Autodesk Inventor part; units mm, degrees
ref_plane "YZ Plane" through (0, 0, 0) normal (1, 0, 0) x (0, 1, 0)
ref_plane "XZ Plane" through (0, 0, 0) normal (0, 1, 0) x (-1, 0, 0)
ref_plane "XY Plane" through (0, 0, 0) normal (0, 0, 1) x (1, 0, 0)
sketch "Sketch1" plane through (0, 0, 0) normal (0, 0, 1) x (1, 0, 0)
  line L0 (0, 0) -> (69.85, 0)
  line L1 (69.85, 0) -> (69.85, 76.2)
  line L2 (0, 76.2) -> (0, 0)
  line L3 (64.77, 76.2) -> (64.77, 5.08)
  line L4 (64.77, 5.08) -> (5.08, 5.08)
  line L5 (5.08, 5.08) -> (5.08, 76.2)
  line L6 (69.85, 76.2) -> (64.77, 76.2)
  line L7 (5.08, 76.2) -> (0, 76.2)
  dimension "d0" = 69.85
  dimension "d1" = 5.08
  dimension "d2" = 5.08
  dimension "d3" = 76.2
extrude "Extrusion1" add sketch "Sketch1" along normal blind 25.4
sketch "Sketch2" plane through (0, 0, 0) normal (0, -1, 0) x (1, 0, 0)
  line L0 (22.225, 38.1) -> (47.625, 38.1)
  line L1 (47.625, 38.1) -> (47.625, -12.7)
  line L2 (47.625, -12.7) -> (22.225, -12.7)
  line L3 (22.225, -12.7) -> (22.225, 38.1)
  line L4 (0, 25.4) -> (69.85, 25.4) construction
  line L5 (0, 25.4) -> (22.225, 38.1) construction
  line L6 (0, 0) -> (69.85, 0) construction
  line L7 (0, 0) -> (22.225, -12.7) construction
  line L8 (47.625, 38.1) -> (69.85, 25.4) construction
  line L9 (47.625, -12.7) -> (69.85, 0) construction
  dimension "d6" = 50.8
  dimension "d7" = 25.4
extrude "Extrusion2" add sketch "Sketch2" against normal up to surface (5.08 mm away)
sketch "Sketch3" plane through (69.85, 0, 0) normal (0, -1, 0) x (1, 0, 0)
  line L0 (-22.225, 38.1) -> (-47.625, 38.1) construction
  line L1 (-47.425, 38.1) -> (-22.425, 38.1) construction
  line L2 (-22.425, 38.1) -> (-22.425, 14.238) construction
  line L3 (-22.425, 14.238) -> (-47.425, 14.238) construction
  line L4 (-47.425, 14.238) -> (-47.425, 38.1) construction
  line L5 (-5.08, 25.4) -> (-22.225, 25.4) construction
  line L6 (-22.225, 25.4) -> (-22.425, 25.4) construction
  line L7 (-69.85, 25.4) -> (-47.625, 25.4) construction
  line L8 (-47.625, 25.4) -> (-47.425, 25.4) construction
  circle A0 centre (-45.425, 16.238) radius 1.25
  circle A1 centre (-24.425, 16.238) radius 1.25
  circle A2 centre (-45.425, 28.738) radius 1.25
  circle A3 centre (-24.425, 28.738) radius 1.25
  line L9 (-39.425, 33.138) -> (-30.425, 33.138)
  line L10 (-30.425, 33.138) -> (-30.425, 24.138)
  line L11 (-30.425, 24.138) -> (-39.425, 24.138)
  line L12 (-39.425, 24.138) -> (-39.425, 33.138)
  line L13 (-39.425, 33.138) -> (-30.425, 24.138) construction
  line L14 (-39.425, 24.138) -> (-30.425, 33.138) construction
  point P0 (-69.85, 0)
  point P1 (-34.925, 28.638)
  dimension "d10" = 23.862
  dimension "d11" = 25
  dimension "d12" = 2.5
  dimension "d13" = 2
  dimension "d14" = 2
  dimension "d15" = 2
  dimension "d16" = 14.5
  dimension "d17" = 9
  dimension "d18" = 9.462
  dimension "d19" = 12.5
extrude "Extrusion3" cut sketch "Sketch3" against normal up to surface (5.08 mm away)
sketch "Sketch4" plane through (0, 0, 0) normal (0, -1, 0) x (1, 0, 0)
  line L0 (22.225, 0) -> (22.225, -12.7) construction
  line L1 (22.225, -12.7) -> (47.625, -12.7) construction
  line L2 (47.625, -12.7) -> (47.625, 12.7) construction
  line L3 (47.625, 12.7) -> (22.225, 12.7) construction
  line L4 (22.225, 12.7) -> (22.225, -12.7) construction
  line L5 (47.625, -12.7) -> (47.625, 0) construction
  line L6 (22.225, 12.7) -> (47.625, -12.7) construction
  line L7 (47.625, 12.7) -> (22.225, -12.7) construction
  line L8 (26.035, 8.89) -> (43.815, 8.89)
  line L9 (43.815, 8.89) -> (43.815, -8.89)
  line L10 (43.815, -8.89) -> (26.035, -8.89)
  line L11 (26.035, -8.89) -> (26.035, 8.89)
  circle A0 centre (24.765, 10.16) radius 1.25
  circle A1 centre (45.085, 10.16) radius 1.25
  circle A2 centre (45.085, -10.16) radius 1.25
  circle A3 centre (24.765, -10.16) radius 1.25
  point P0 (0, 0)
  dimension "d22" = 2.5
  dimension "d23" = 20.32
  dimension "d24" = 17.78
extrude "Extrusion4" cut sketch "Sketch4" against normal up to surface (5.08 mm away)
sketch "Sketch5" plane through (0, 0, 0) normal (-1, 0, 0) x (0, 0, 1)
  line L0 (0, 76.2) -> (25.4, 76.2) construction
  line L1 (0, 76.2) -> (0, 5.08) construction
  line L2 (25.4, 76.2) -> (0, 76.2) construction
  line L3 (0, 76.2) -> (0, 50.8) construction
  line L4 (0, 50.8) -> (25.4, 50.8) construction
  line L5 (25.4, 50.8) -> (25.4, 76.2) construction
  line L6 (25.4, 76.2) -> (0, 50.8) construction
  line L7 (25.4, 50.8) -> (0, 76.2) construction
  arc A0 (14.4861, 60.875) -> (10.9139, 60.875) centre (12.7, 63.5) ccw construction
  line L8 (14.4861, 60.875) -> (10.9139, 60.875) construction
  line L9 (10.8534, 60.675) -> (14.5466, 60.675)
  arc A1 (14.5466, 60.675) -> (10.8534, 60.675) centre (12.7, 63.5) ccw
  point P0 (0, 0)
  dimension "d27" = 25.4
  dimension "d28" = 6.35
  dimension "d29" = 5.8
  dimension "d54" = 0.2
extrude "Extrusion5" cut sketch "Sketch5" against normal up to surface (5.08 mm away)
sketch "Sketch6" plane through (69.85, 0, 0) normal (1, 0, 0) x (0, 0, -1)
  line L0 (-25.4, 76.2) -> (-25.4, 0) construction
  line L1 (-25.4, 76.2) -> (0, 50.8) construction
  line L2 (0, 76.2) -> (0, 0) construction
  line L3 (0, 76.2) -> (-25.4, 76.2) construction
  line L4 (0, 76.2) -> (-25.4, 50.8) construction
  line L5 (-25.4, 0) -> (-25.4, 76.2) construction
  line L6 (-25.4, 50.8) -> (0, 50.8) construction
  line L7 (-25.4, 5.08) -> (-25.4, 76.2)
  circle A0 centre (-12.7, 63.5) radius 2.6035
  dimension "d52" = 25.4
  dimension "d53" = 5.207
extrude "Extrusion6" cut sketch "Sketch6" against normal up to surface (5.08 mm away)
fillet "Fillet1" radius 2 4 edges at (47.625, 2.54, 38.1) (22.225, 2.54, 38.1) (22.225, 2.54, -12.7) (47.625, 2.54, -12.7)
fillet "Fillet2" radius 6.35 4 edges at (67.31, 76.2, 25.4) (67.31, 76.2, 0) (2.54, 76.2, 25.4) (2.54, 76.2, 0)
chamfer "Chamfer1" distance 6.35 angle 45 4 edges at (0, 0, 12.7) (5.08, 5.08, 12.7) (69.85, 0, 12.7) (64.77, 5.08, 12.7)
sketch "Sketch7" plane through (0, 76.2, 6.35) normal (-1, 0, 0) x (0, 0, 1)
  line L0 (12.7, -22.225) -> (0, -22.225)
  line L1 (0, -22.225) -> (0, -69.85)
  line L2 (0, -69.85) -> (12.7, -69.85)
  line L3 (12.7, -69.85) -> (12.7, -22.225)
  line L4 (-6.35, -6.35) -> (-6.35, -69.85)
  line L5 (19.05, -69.85) -> (-6.35, -69.85)
  line L6 (19.05, -6.35) -> (19.05, -69.85)
  arc A0 (8.975, -10.9139) -> (8.975, -14.4861) centre (6.35, -12.7) ccw
  point P0 (-6.35, -76.2)
  dimension "d42" = 6.35
  dimension "d43" = 0
  dimension "d44" = 6.35
  dimension "d46" = 6.35
extrude "Extrusion7" cut sketch "Sketch7" against normal through all
chamfer "Chamfer2" distance 3.175 angle 45 8 edges at (64.77, 6.35, 19.05) (64.77, 6.35, 6.35) (67.31, 53.975, 6.35) (67.31, 53.975, 19.05) (5.08, 6.35, 6.35) (5.08, 6.35, 19.05) (2.54, 53.975, 19.05) (2.54, 53.975, 6.35)
fillet "Fillet3" radius 3.175 4 edges at (26.035, 2.54, 8.89) (26.035, 2.54, -8.89) (43.815, 2.54, -8.89) (43.815, 2.54, 8.89)
sketch "Sketch8" plane through (0, 76.2, 6.35) normal (-1, 0, 0) x (0, 0, 1)
  arc A0 (8.1966, -15.525) -> (4.5034, -15.525) centre (6.35, -12.7) ccw
  line L0 (8.1966, -15.525) -> (4.5034, -15.525)
  arc A1 (8.6238, -17.125) -> (4.0762, -17.125) centre (6.35, -12.7) ccw
  line L1 (8.6238, -17.125) -> (4.0762, -17.125)
  point P0 (-6.35, -76.2)
  dimension "d56" = 1.6
extrude "Extrusion8" add sketch "Sketch8" along normal blind 4.525
sketch "Sketch9" plane through (5.08, 76.2, 19.05) normal (1, 0, 0) x (0, 0, -1)
  line L0 (8.1966, -15.525) -> (4.5034, -15.525)
  arc A0 (8.1966, -15.525) -> (4.5034, -15.525) centre (6.35, -12.7) ccw
  line L1 (4.0762, -17.125) -> (8.6238, -17.125)
  arc A1 (8.6238, -17.125) -> (4.0762, -17.125) centre (6.35, -12.7) ccw
  point P0 (19.05, -76.2)
  dimension "d59" = 1.6
extrude "Extrusion9" add sketch "Sketch9" along normal blind 5.4
sketch "Sketch10" plane through (69.85, 76.2, 19.05) normal (1, 0, 0) x (0, 0, -1)
  circle A0 centre (6.35, -12.7) radius 2.6035
  circle A1 centre (6.35, -12.7) radius 4.2035
  point P0 (19.05, -76.2)
  dimension "d62" = 1.6
extrude "Extrusion10" add sketch "Sketch10" along normal blind 2.54
properties part number "HoseMount"
Check sheet for the modelled part. Datum: model origin and axes. Units: mm. A direction names the side the tool comes from. Give positions to 0.01 mm unless a question says otherwise; leave off trailing zeros. Loops run counter-clockwise (first coordinate to the right, second up) from the corner with the lowest first, then second, coordinate; pieces in that order, holes last. Notation, with made-up numbers: (10, 23.5) - (14, 23.5) arc R17 ccw to (14, 47.5) - close; hole circle Ø9 at (18, -9). An arc over 180 degrees is marked (long way). One line per question, with ' | ' between items. Start each with the question number.
1. Material ranges on line 1 along X through (y, z) = (1, -10) (3 decimals); line 2 along Z through (x, y) = (0.5, 63.5); line 3 along X through (y, z) = (48.5, 22), recorded low to high. Write a range as [from, to].
2. Draft check along X on faces 6 (the flat face through (10.48, 65, 16)), 7 (the cylindrical face through (22.795, 2.576, 37.499)), 8 (the flat face through (35, 3, 8.89)), 9 (the flat face through (65.828, 7.96, 17.485)). Enter one of: released by +X, released by -X, zero draft, split by the parting line, or undercut.
3. Gauge pin test, flat ends, axial feed: pin 1 Ø6 at (x, z) = (39, 27) entering from +Y; pin 2 Ø3 at (y, z) = (12, -1) entering from +X; pin 3 Ø2.5 at (y, z) = (2, 30.5) entering from +X (3 decimals); pin 4 Ø3 at (x, z) = (45.085, 10.16) entering from -Y. Record the tip position at first contact, or that the pin passes through.
4. Cross-section at C-C, the plane z = 12.7. Give the number of separate pieces and of enclosed holes in the cut face, plus the area to 3 significant figures.
5. Cross-section at A-A, the plane y = 28. Enter the section's corners in (x, z).
6. Set-up check for faces 1 (the flat face through (4, 27, 0)), 2 (the flat face through (39.425, 3, 29)), 3 (the cylindrical face through (3.083, 66.873, 12.579)), 4 (the flat face through (64.77, 59, 13)), 5 (the flat face through (68, 30, 6.35)): record each of +Z, -Z, +X, -X, +Y, -Y from which the full face is reachable in a straight line by a thin tool's end or side.
7. Cross-section at B-B, the plane x = 36. Enter the section's corners in (y, z).
Check result:
1) line 1: x = [22.225, 23.525], [26.005, 43.845], [46.325, 47.625] | line 2: z = [0, 9.33], [16.07, 25.4] | line 3: x = [0, 5.08], [64.77, 69.85]
2) face 6: undercut | face 7: released by -X | face 8: undercut | face 9: zero draft
3) pin 1: stops at y = 5.08 | pin 2: stops at x = 69.85 | pin 3: stops at x = 47.625 | pin 4: stops at y = 0
4) separate pieces: 5 | enclosed holes: 0 | area: 550 mm2
5) outline: (0, 0) - (5.08, 0) - (5.08, 6.35) - (0, 6.35) - close; (0, 19.05) - (5.08, 19.05) - (5.08, 25.4) - (0, 25.4) - close; (64.77, 0) - (69.85, 0) - (69.85, 6.35) - (64.77, 6.35) - close; (64.77, 19.05) - (69.85, 19.05) - (69.85, 25.4) - (64.77, 25.4) - close
6) face 1: -Z, -X, +Y, -Y | face 2: +Y, -Y | face 3: -X | face 4: +Z, -Z, +Y | face 5: +X, -X
7) outline: (0, -12.7) - (5.08, -12.7) - (5.08, -8.89) - (0, -8.89) - close; (0, 8.89) - (5.08, 8.89) - (5.08, 24.14) - (0, 24.14) - close; (0, 33.14) - (5.08, 33.14) - (5.08, 38.1) - (0, 38.1) - close
